```python
from build123d import *

# Parameters (mm, degrees)
EXTRUDE_1_DEPTH        = 19.9
EXTRUDE_1_DEPTH_BACK   = 19.9
EXTRUDE_1_2_DEPTH      = 19.9
EXTRUDE_1_2_DEPTH_BACK = 19.9
EXTRUDE_2_DEPTH        = 12.1
EXTRUDE_4_DEPTH        = 12.1
EXTRUDE_5_DEPTH        = 12.1
SKETCH_4_R             = 2.1
CUT_EXTRUDE_1_DEPTH    = 74.077252942
CUT_EXTRUDE_2_DEPTH    = 3.5
SKETCH_9_R             = 1
EXTRUDE_6_DEPTH        = 12
DRAFT_START            = -52
DRAFT_3_DEPTH          = 11.517207928
DRAFT_START_2          = 40.482792072
DRAFT_5_DEPTH          = 11.517207928
SKETCH_10_R            = 2
CUT_EXTRUDE_3_DEPTH    = 77.242064239


with BuildPart() as part:
    # Sketch 1 → Extrude 1 (new, two sides: drawn at the far end of the back side and taken through both)
    with BuildSketch(Plane(origin=(0, 0, 0), x_dir=(1, 0, 0), z_dir=(0, 1, 0)).offset(-EXTRUDE_1_DEPTH_BACK)):
        with BuildLine():
            Line((38.470009909, -33.482209271), (32.917480236, -29.196566492))
            Line((32.917480236, -29.196566492), (33.95705193, -38.051525912))
            ThreePointArc((33.95705193, -38.051525912), (36.285527215, -35.837975874), (38.470009909, -33.482209271))
        make_face()
    extrude(amount=EXTRUDE_1_DEPTH + EXTRUDE_1_DEPTH_BACK)



with BuildPart() as body_2:
    # Sketch 1 → Extrude 1 2 (new, two sides: drawn at the far end of the back side and taken through both)
    with BuildSketch(Plane(origin=(0, 0, 0), x_dir=(1, 0, 0), z_dir=(0, 1, 0)).offset(-EXTRUDE_1_2_DEPTH_BACK)):
        with BuildLine():
            Line((-32.917480236, -29.196566492), (-38.470009909, -33.482209271))
            ThreePointArc((-38.470009909, -33.482209271), (-36.064957562, -36.059933944), (-33.487567945, -38.465345353))
            Line((-33.487567945, -38.465345353), (-32.917480236, -29.196566492))
        make_face()
    extrude(amount=EXTRUDE_1_2_DEPTH + EXTRUDE_1_2_DEPTH_BACK)


with BuildPart() as part_1:
    add(part.part)

    add(body_2.part)  # Extrude 2 merges body 2
    # Sketch 2 → Extrude 2 (add)
    with BuildSketch(Plane(origin=(0, 19.9, 0), x_dir=(1, 0, 0), z_dir=(0, 1, 0))):
        with BuildLine():
            Line((-32.917480236, -29.196566492), (-38.470009909, -33.482209271))
            ThreePointArc((-38.470009909, -33.482209271), (-36.064957562, -36.059933944), (-33.487567945, -38.465345353))
            ThreePointArc((-33.487567945, -38.465345353), (0.312914422, -50.999040036), (33.95705193, -38.051525912))
            ThreePointArc((33.95705193, -38.051525912), (36.285527215, -35.837975874), (38.470009909, -33.482209271))
            Line((38.470009909, -33.482209271), (32.917480236, -29.196566492))
            Line((32.917480236, -29.196566492), (33.669275707, -35.60027912))
            ThreePointArc((33.669275707, -35.60027912), (0.231869073, -48.999451392), (-33.33084903, -35.917328727))
            Line((-33.33084903, -35.917328727), (-32.917480236, -29.196566492))
        make_face()
    extrude_2 = extrude(amount=EXTRUDE_2_DEPTH)

    # Mirror 4: Extrude 2 across plane
    add(extrude_2.mirror(Plane.ZX))

    # Sketch 5 → Extrude 4 (add)
    with BuildSketch(Plane(origin=(0, 32, 0), x_dir=(1, 0, 0), z_dir=(0, 1, 0))):
        with BuildLine():
            Line((-18.169872981, -41.47114317), (-26.830127019, -36.47114317))
            Line((-26.830127019, -36.47114317), (-30.324983414, -38.488899451))
            ThreePointArc((-30.324983414, -38.488899451), (-24.5, -42.435244785), (-18.169872981, -45.506655731))
            Line((-18.169872981, -45.506655731), (-18.169872981, -41.47114317))
        make_face()
        with BuildLine():
            Line((26.830127019, -36.47114317), (30.324983414, -38.488899451))
            ThreePointArc((30.324983414, -38.488899451), (24.5, -42.435244785), (18.169872981, -45.506655731))
            Line((18.169872981, -45.506655731), (18.169872981, -41.47114317))
            Line((18.169872981, -41.47114317), (26.830127019, -36.47114317))
        make_face()
    extrude(amount=-EXTRUDE_4_DEPTH)

    # Sketch 6 → Extrude 5 (add)
    with BuildSketch(Plane.XZ.offset(32)):
        with BuildLine():
            Line((18.169872981, 41.47114317), (18.169872981, 45.506655731))
            ThreePointArc((18.169872981, 45.506655731), (24.5, 42.435244785), (30.324983414, 38.488899451))
            Line((30.324983414, 38.488899451), (26.830127019, 36.47114317))
            Line((26.830127019, 36.47114317), (18.169872981, 41.47114317))
        make_face()
        with BuildLine():
            Line((-26.830127019, 36.47114317), (-30.324983414, 38.488899451))
            ThreePointArc((-30.324983414, 38.488899451), (-24.5, 42.435244785), (-18.169872981, 45.506655731))
            Line((-18.169872981, 45.506655731), (-18.169872981, 41.47114317))
            Line((-18.169872981, 41.47114317), (-26.830127019, 36.47114317))
        make_face()
    extrude(amount=-EXTRUDE_5_DEPTH)

    # Sketch 4 → Cut-Extrude 1 (cut, through all)
    with BuildSketch(Plane(origin=(-25.5, 0, 44.167295593), x_dir=(0.8660254037844417, 0, 0.4999999999999947), z_dir=(-0.4999999999999947, 0, 0.8660254037844417))):
        with Locations((0, -26)):
            Circle(SKETCH_4_R)
        with Locations((0, 26)):
            Circle(SKETCH_4_R)
    cut_extrude_1 = extrude(amount=-CUT_EXTRUDE_1_DEPTH, mode=Mode.SUBTRACT)

    # Mirror 5: Cut-Extrude 1 across plane
    add(cut_extrude_1.mirror(Plane(origin=(0, 0, 0), x_dir=(0, 0, 1), z_dir=(1, 0, 0))), mode=Mode.SUBTRACT)

    # Sketch 7 → Cut-Extrude 2 (cut)
    with BuildSketch(Plane(origin=(-22.5, 0, 38.97114317), x_dir=(-0.866025403784438, 0, -0.5000000000000011), z_dir=(0.5000000000000011, 0, -0.8660254037844382))):
        Polygon((4.099186911, 26), (2.049593456, 29.55), (-2.049593456, 29.55), (-4.099186911, 26), (-2.049593456, 22.45), (2.049593456, 22.45), align=None)
        Polygon((2.049593456, -22.45), (4.099186911, -26), (2.049593456, -29.55), (-2.049593456, -29.55), (-4.099186911, -26), (-2.049593456, -22.45), align=None)
    cut_extrude_2 = extrude(amount=-CUT_EXTRUDE_2_DEPTH, mode=Mode.SUBTRACT)

    # Mirror 7: Cut-Extrude 2 across plane
    add(cut_extrude_2.mirror(Plane(origin=(0, 0, 0), x_dir=(0, 0, 1), z_dir=(1, 0, 0))), mode=Mode.SUBTRACT)

    # Sketch 9 → Extrude 6 (add)
    # profile 1 of 2: a face of its own
    with BuildSketch(Plane(origin=(0, -0.85, 0), x_dir=(-1, 0, 0), z_dir=(0, -1, 0))):
        with BuildLine():
            ThreePointArc((-44.691496308, -24.569699993), (-41.818862185, -29.192169593), (-38.470009909, -33.482209271))
            Line((-38.470009909, -33.482209271), (-32.917480236, -29.196566492))
            Line((-32.917480236, -29.196566492), (-32.917480236, -25))
            ThreePointArc((-32.917480236, -25), (-34.921838684, -21.485997557), (-38.966789918, -21.422472216))
            Line((-38.966789918, -21.422472216), (-44.691496308, -24.569699993))
        make_face()
        with Locations(Location((-37, -25, 0), (0, 0, 90))):
            Circle(SKETCH_9_R, mode=Mode.SUBTRACT)
    # profile 2 of 2: a face of its own
    with BuildSketch(Plane(origin=(0, -0.85, 0), x_dir=(-1, 0, 0), z_dir=(0, -1, 0))):
        with BuildLine():
            ThreePointArc((38.470009909, -33.482209271), (41.818862185, -29.192169593), (44.691496308, -24.569699993))
            Line((44.691496308, -24.569699993), (38.966789918, -21.422472216))
            ThreePointArc((38.966789918, -21.422472216), (34.921838684, -21.485997557), (32.917480236, -25))
            Line((32.917480236, -25), (32.917480236, -29.196566492))
            Line((32.917480236, -29.196566492), (38.470009909, -33.482209271))
        make_face()
        with Locations(Location((37, -25, 0), (0, 0, 90))):
            Circle(SKETCH_9_R, mode=Mode.SUBTRACT)
    extrude(amount=EXTRUDE_6_DEPTH)

    # Draft 3: read off the stored shape, not the designer's step
    # Draft 3 outline → Draft 3 (cut)
    with BuildSketch(Plane(origin=(0, 0, 0), x_dir=(0.6110056787485416, 0, 0.7916262126389156), z_dir=(0.7916262126389156, 0, -0.611005678748542)).offset(DRAFT_START)):
        Polygon((-9, 0.85), (3, 12.85), (-9, 12.85), align=None)
    extrude(amount=DRAFT_3_DEPTH, mode=Mode.SUBTRACT)

    # Draft 5: read off the stored shape, not the designer's step
    # Draft 5 outline → Draft 5 (cut)
    with BuildSketch(Plane(origin=(0, 0, 0), x_dir=(0.6110056787485442, 0, -0.7916262126389138), z_dir=(0.7916262126389138, 0, 0.6110056787485444)).offset(DRAFT_START_2)):
        Polygon((9, -0.85), (-3, -12.85), (9, -12.85), align=None)
    extrude(amount=DRAFT_5_DEPTH, mode=Mode.SUBTRACT)

    # Sketch 10 → Cut-Extrude 3 (cut, through all)
    with BuildSketch(Plane(origin=(0, -2.85, 0), x_dir=(1, 0, 0), z_dir=(0, 1, 0))):
        with Locations(Location((-37, -25, 0), (0, 0, 270))):
            Circle(SKETCH_10_R)
        with Locations(Location((37, -25, 0), (0, 0, 52.337744339))):
            Circle(SKETCH_10_R)
    extrude(amount=-CUT_EXTRUDE_3_DEPTH, mode=Mode.SUBTRACT)


solid = part_1.part
```
Design review of the part built by this model. Coordinates are the model's own, in mm. A direction names the side the tool comes from. Round coordinates to 2 decimals unless told otherwise and drop trailing zeros. Write each loop counter-clockwise with the first axis right and the second up, starting at its lowest first coordinate (ties: lowest second). Pieces come first, ordered by that corner, then holes. Notation, with made-up numbers: (54, 45) -> (94, 45) arc R22 cw to (94, 78) -> close; hole circle Ø7 at (89, 81.5). An arc over 180 degrees is marked (long way). Answer in a Markdown table with one row per item.
Q1. Take a section at A-A, the plane x = -17. State the section outline as (y, z) points, then the cut area to 3 significant figures.
The answers:
| item | result |
|---|---|
| outline | (-32, 45.96) -> (-19.9, 45.96) -> (-19.9, 48.08) -> (-32, 48.08) -> close; (19.9, 45.96) -> (32, 45.96) -> (32, 48.08) -> (19.9, 48.08) -> close |
| area | 51.5 mm² |
Q2. Draft analysis for pull direction Y (two halves, no side actions). For faces 1 (the face through (0, 32, 50)), 2 (the face through (18.17, -26, 43)), 3 (the face through (23, -29.55, 40)), state which applies: +Y half, -Y half, draft (parallel to the pull), parting line (faces both ways), or undercut.
The answers:
| item | result |
|---|---|
| face 1 | +Y half |
| face 2 | draft |
| face 3 | undercut |
Q3. Take a section at C-C, the plane y = 2. State the section outline as (x, z) points, then the cut area to 3 significant figures.
The answers:
| item | result |
|---|---|
| outline | (-38.47, 33.48) -> (-32.92, 29.2) -> (-33.49, 38.47) arc R51 ccw to start; (32.92, 29.2) -> (38.47, 33.48) arc R51 ccw to (33.96, 38.05) -> close |
| area | 47.9 mm² |
Q4. To check wall thickness, follow L1, parallel to Y at x = -24, z = 40.5; L2, parallel to Y at x = 2, z = 49; L3, parallel to X at y = 24.5, z = 37. State the ranges of each line that lie inside material, in increasing order. Write a range as [from, to].
The answers:
| item | result |
|---|---|
| L1 | [-32, -29.55], [-22.45, -19.9], [19.9, 22.45], [29.55, 32] |
| L2 | [-32, -19.9], [19.9, 32] |
| L3 | [-35.1, -32.12], [-27.75, -25.91], [25.91, 27.75], [32.12, 35.1] |
Q5. Take a section at B-B, the plane z = 31.5. State the section outline as (x, y) points.
The answers:
| item | result |
|---|---|
| outline | (-40.11, -10.28) -> (-35.9, -12.85) -> (-35.9, -32) -> (-33.06, -32) -> (-33.06, 32) -> (-35.9, 32) -> (-35.9, -0.85) -> (-40.11, -0.85) -> close; (33.19, -32) -> (35.9, -32) -> (35.9, -12.85) -> (40.11, -10.28) -> (40.11, -0.85) -> (35.9, -0.85) -> (35.9, 32) -> (33.19, 32) -> close |
Q6. Take a section at D-D, the plane z = 46.5. State the section outline as (x, y) points, then the cut area to 3 significant figures.
The answers:
| item | result |
|---|---|
| outline | (-20.95, -32) -> (-15.45, -32) -> (-15.45, -19.9) -> (-20.95, -19.9) -> close; (-20.95, 19.9) -> (-15.45, 19.9) -> (-15.45, 32) -> (-20.95, 32) -> close; (15.45, -32) -> (20.95, -32) -> (20.95, -19.9) -> (15.45, -19.9) -> close; (15.45, 19.9) -> (20.95, 19.9) -> (20.95, 32) -> (15.45, 32) -> close |
| area | 266 mm² |
Q7. For faces 4 (the face through (23, 29.55, 40)), 5 (the face through (20.713, -27.8, 41.995)), 6 (the face through (-22.439, 22.001, 39.006)), list the 3-axis set-ups (+Z, -Z, +X, -X, +Y, -Y) from which the entire face can be reached by the end or side of a thin tool; tool diameter is ignored.
The answers:
| item | result |
|---|---|
| face 4 | none |
| face 5 | -Z |
| face 6 | -Z, +Y, -Y |
Q8. Clearance check with flat-ended pins moving along their axes: pin 1 Ø8 at (x, y) = (-22, -23) entering from -Z; pin 2 Ø2 at (y, z) = (-9, 34) entering from -X; pin 3 Ø2.5 at (x, z) = (-37, 25) entering from -Y. State where each tip first meets the part, or that it passes through.
The answers:
| item | result |
|---|---|
| pin 1 | z = 36.95 |
| pin 2 | x = -38.88 |
| pin 3 | y = -2.85 |
